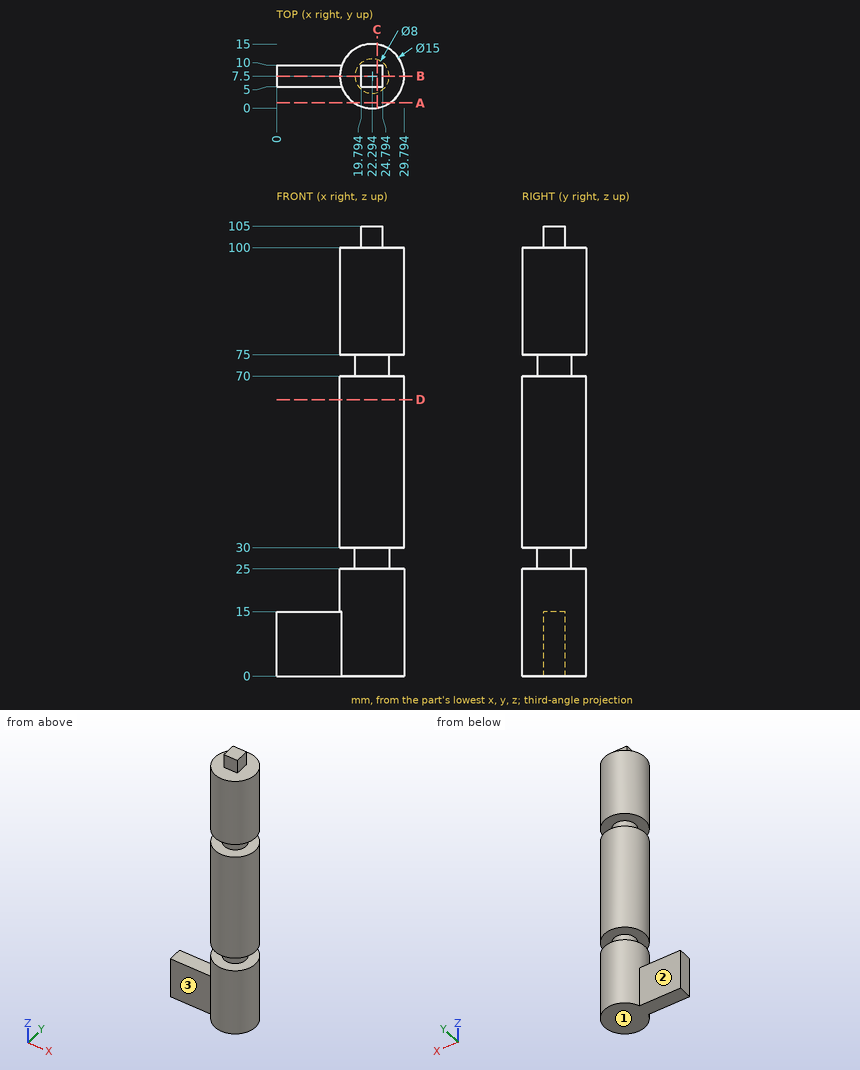
Can you work these out from the drawing? Everything is in mm from the part's minimum corner. A direction names the side the tool comes from. Coordinates: 2 decimals unless noted, no trailing zeros. Loops run counter-clockwise (first coordinate to the right, second up) from the corner with the lowest first, then second, coordinate; pieces in that order, holes last. Notation, with made-up numbers: (88.25, -30.75) - (94.25, -30.75) arc R28 ccw to (94.25, -2.75) - close; hole circle Ø2 at (71, 19.5). An arc over 180 degrees is marked (long way). Use a Markdown table: item, result.
Item 1: If I drill on probe 1 along Z at (x, y) = (20, 3.75); probe 2 along X at (y, z) = (8, 9); probe 3 along Y at (x, z) = (22, 79) (1 decimal), over which ranges is the centre line in solid material (lowest first)? Write a range as from..to.
Numbers:
| item | result |
|---|---|
| probe 1 | z = 0..25, 30..70, 75..100 |
| probe 2 | x = 0..29.78 |
| probe 3 | y = 0..15 |
Item 2: I want a section at A-A on y = 1.25. Please give me the cut outline in (x, z), and give its area (3 significant figures).
Numbers:
| item | result |
|---|---|
| outline | (18.15, 0) - (26.44, 0) - (26.44, 25) - (18.15, 25) - close; (18.15, 30) - (26.44, 30) - (26.44, 70) - (18.15, 70) - close; (18.15, 75) - (26.44, 75) - (26.44, 100) - (18.15, 100) - close |
| area | 746 mm2 |
Item 3: I want a section at D-D on z = 64.5. Please give me the cut outline in (x, y) (1 decimal), and give its area (3 significant figures).
Numbers:
| item | result |
|---|---|
| outline | circle Ø15 at (22.3, 7.5) |
| area | 177 mm2 |
Item 4: I want a section at B-B on y = 7.5. Please give me the cut outline in (x, z) (1 decimal), and give its area (3 significant figures).
Numbers:
| item | result |
|---|---|
| outline | (0, 0) - (29.8, 0) - (29.8, 25) - (26.3, 25) - (26.3, 30) - (29.8, 30) - (29.8, 70) - (26.3, 70) - (26.3, 75) - (29.8, 75) - (29.8, 100) - (24.8, 100) - (24.8, 105) - (19.8, 105) - (19.8, 100) - (14.8, 100) - (14.8, 75) - (18.3, 75) - (18.3, 70) - (14.8, 70) - (14.8, 30) - (18.3, 30) - (18.3, 25) - (14.8, 25) - (14.8, 15) - (0, 15) - close |
| area | 1,680 mm2 |
Item 5: I want a section at C-C on x = 23.5. Please give me the cut outline in (y, z) (1 decimal).
Numbers:
| item | result |
|---|---|
| outline | (0.1, 0) - (14.9, 0) - (14.9, 25) - (11.3, 25) - (11.3, 30) - (14.9, 30) - (14.9, 70) - (11.3, 70) - (11.3, 75) - (14.9, 75) - (14.9, 100) - (10, 100) - (10, 105) - (5, 105) - (5, 100) - (0.1, 100) - (0.1, 75) - (3.7, 75) - (3.7, 70) - (0.1, 70) - (0.1, 30) - (3.7, 30) - (3.7, 25) - (0.1, 25) - close |
Item 6: Will these pins go through, and if not, where does the flat tip stop? pin 1 (2.5 mm diameter, centred on x = 22, z = 103.5, fed in from +Y); pin 2 (16.5 mm diameter, centred on x = 6.5, z = 7.5, fed in from -Y); pin 3 (1.5 mm diameter, centred on x = 9, y = 8, fed in from +Z).
Numbers:
| item | result |
|---|---|
| pin 1 | stops at y = 10 |
| pin 2 | stops at y = 5 |
| pin 3 | stops at z = 15 |
Item 7: For the marked faces 1, 2 and 3, which set-ups out of +Z, -Z, +X, -X, +Y, -Y let a thin tool reach every point of the face, with its end or its side?
Numbers:
| item | result |
|---|---|
| face 1 | -Z, +X, -X, +Y, -Y |
| face 2 | +Z, -Z, -X, +Y |
| face 3 | +Z, -Z, -X, -Y |
